The drawing under review shows one solid part. Ordinate dimensions are in mm from its lowest x, y, z. A direction names the side the tool comes from. Coordinates: 2 decimals unless noted, no trailing zeros. Loops run counter-clockwise (first coordinate to the right, second up) from the corner with the lowest first, then second, coordinate; pieces in that order, holes last. Notation, with made-up numbers: (28.5, -3.5) - (75.5, -3.5) arc R22 cw to (75.5, 25.5) - close; hole circle Ø10 at (41.25, 5.5). An arc over 180 degrees is marked (long way). Answer as a JSON object with one key per item and string values. Group by question number.
Item 1: We need section C-C (z = 2.75). Give the boundary of the cut face in (x, y), then the cut area to 3 significant figures.
Item 2: Tool access review of the marked faces 1 and 2: name each direction out of +Z, -Z, +X, -X, +Y, -Y from which nothing blocks a thin tool from reaching the whole face with its end or side.
Item 3: To check wall thickness, follow line 1 (X direction, y = 42, z = 12); line 2 (X direction, y = 6, z = 3.5); line 3 (Z direction, x = 70, y = 16.5). State the ranges of each line that lie inside material, in increasing order.
Item 4: Clearance check with flat-ended pins moving along their axes: pin 1 (3.5 mm diameter, centred on x = 136, y = 32.5, fed in from -Z); pin 2 (10 mm diameter, centred on y = 23, z = 23.5, fed in from +X); pin 3 (2 mm diameter, centred on y = 26, z = 2.5, fed in from -X); pin 4 (2 mm diameter, centred on y = 28.5, z = 2, fed in from +X). State where each tip first meets the part, or that it passes through.
Item 5: We need section B-B (y = 19). Give the boundary of the cut face in (x, z), then the cut area to 3 significant figures.
Item 6: Mouldability with a two-part tool opening along X and no side actions: class the marked faces 3, 4 and 5 as released by +X, released by -X, zero draft, split by the parting line, or undercut.
Item 7: We need section D-D (x = 33). Give the boundary of the cut face in (y, z), then the cut area to 3 significant figures.
Item 8: We need section A-A (z = 17). Give the boundary of the cut face in (x, y), then the cut area to 3 significant figures.
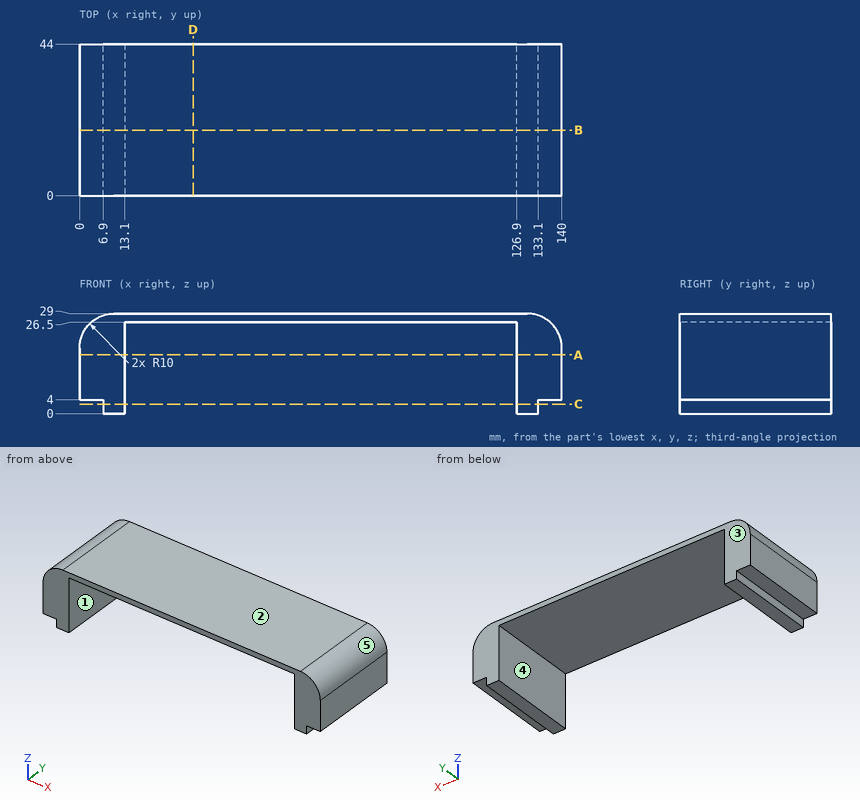
Check sheet entries:
{
 "1": {"outline": "(6.9, 0) - (13.1, 0) - (13.1, 44) - (6.9, 44) - close; (126.9, 0) - (133.1, 0) - (133.1, 44) - (126.9, 44) - close", "area": "546 mm2"},
 "2": {"face 1": "-Z, +Y, -Y", "face 2": "+Z, +X, -X, +Y, -Y"},
 "3": {"line 1": "x = 0 to 13.1, 126.9 to 140", "line 2": "x = 6.9 to 13.1, 126.9 to 133.1", "line 3": "z = 26.5 to 29"},
 "4": {"pin 1": "stops at z = 4", "pin 2": "stops at x = 140", "pin 3": "stops at x = 6.9", "pin 4": "stops at x = 133.1"},
 "5": {"outline": "(0, 4) - (6.9, 4) - (6.9, 0) - (13.1, 0) - (13.1, 26.5) - (126.9, 26.5) - (126.9, 0) - (133.1, 0) - (133.1, 4) - (140, 4) - (140, 19) arc R10 ccw to (130, 29) - (10, 29) arc R10 ccw to (0, 19) - close", "area": "946 mm2"},
 "6": {"face 3": "zero draft", "face 4": "undercut", "face 5": "released by +X"},
 "7": {"outline": "(0, 26.5) - (44, 26.5) - (44, 29) - (0, 29) - close", "area": "110 mm2"},
 "8": {"outline": "(0, 0) - (13.1, 0) - (13.1, 44) - (0, 44) - close; (126.9, 0) - (140, 0) - (140, 44) - (126.9, 44) - close", "area": "1,150 mm2"}
}
